```python
from build123d import *

# Parameters (mm, degrees)
SKETCH1_W           = 175
SKETCH1_H           = 150
BOSS_EXTRUDE1_DEPTH = 15
CUT_EXTRUDE1_DEPTH  = 231.976189249
SKETCH3_W           = 50
SKETCH3_H           = 30
BOSS_EXTRUDE2_DEPTH = 50
SKETCH4_W           = 40.3
SKETCH4_H           = 20.3
BOSS_EXTRUDE3_DEPTH = 25
SKETCH5_R           = 5
CUT_EXTRUDE3_DEPTH  = 206.184770127
SKETCH7_R           = 6
CUT_EXTRUDE5_DEPTH  = 248.25951426
SKETCH8_R           = 12.5
CUT_EXTRUDE6_DEPTH  = 12.5


with BuildPart() as part:
    # Sketch1 → Boss-Extrude1 (new body)
    with BuildSketch(Plane(origin=(0, 0, 0), x_dir=(1, 0, 0), z_dir=(0, 1, 0))):
        with Locations((87.5, 75)):
            Rectangle(SKETCH1_W, SKETCH1_H)
    extrude(amount=BOSS_EXTRUDE1_DEPTH)

    # Sketch2 → Cut-Extrude1 (cut, through all)
    with BuildSketch(Plane(origin=(175, 0, 0), x_dir=(0, 0, -1), z_dir=(1, 0, 0))):
        Polygon((150, 15), (0, 5), (0, 15), align=None)
    extrude(amount=-CUT_EXTRUDE1_DEPTH, mode=Mode.SUBTRACT)

    # Sketch3 → Boss-Extrude2 (add)
    with BuildSketch(Plane(origin=(0, 4.977876106, 0.331858407), x_dir=(1, 0, 0), z_dir=(0, 0.997785157856609, 0.06651901052377394))):
        with Locations((87.5, 135.665558836)):
            Rectangle(SKETCH3_W, SKETCH3_H)
    extrude(amount=BOSS_EXTRUDE2_DEPTH)

    # Sketch4 → Boss-Extrude3 (add)
    with BuildSketch(Plane(origin=(0, 54.867133999, 3.657808933), x_dir=(1, 0, 0), z_dir=(0, 0.997785157856609, 0.0665190105237739))):
        with Locations((87.5, 135.665558836)):
            Rectangle(SKETCH4_W, SKETCH4_H)
    extrude(amount=BOSS_EXTRUDE3_DEPTH)

    # Sketch5 → Cut-Extrude3 (cut, through all)
    with BuildSketch(Plane.ZY.offset(-67.35)):
        with Locations((-130.875784474, 76.363787208)):
            Circle(SKETCH5_R)
    extrude(amount=-CUT_EXTRUDE3_DEPTH, mode=Mode.SUBTRACT)

    # Sketch7 → Cut-Extrude5 (cut, through all)
    with BuildSketch(Plane.XZ):
        with Locations(Location((87.5, -131.674049474, 0), (0, 0, 270))):
            Circle(SKETCH7_R)
    extrude(amount=-CUT_EXTRUDE5_DEPTH, mode=Mode.SUBTRACT)

    # Sketch8 → Cut-Extrude6 (cut)
    with BuildSketch(Plane.XZ):
        with Locations(Location((87.5, -131.674049474, 0), (0, 0, 270))):
            Circle(SKETCH8_R)
    extrude(amount=-CUT_EXTRUDE6_DEPTH, mode=Mode.SUBTRACT)


solid = part.part
```
CAD build for the part. Positions are in the model's coordinates, mm. A direction names the side the tool comes from. Coordinates: 2 decimals unless noted, no trailing zeros. Write each loop counter-clockwise with the first axis right and the second up, starting at its lowest first coordinate (ties: lowest second). Pieces come first, ordered by that corner, then holes. Notation, with made-up numbers: (74.25, -17) -> (110.25, -17) arc R17 ccw to (110.25, 9) -> close; hole circle Ø5 at (-8, -34). An arc over 180 degrees is marked (long way). Return JSON: item names as keys, results as strings. Group by question number.
Q1. Cut at C-C, the plane z = -86. Give the cut face in (x, y), then the cut area to 3 significant figures.
Q2. Drill centre lines: line 1 (X direction, y = 41, z = -121); line 2 (X direction, y = 51, z = -127.5); line 3 (Y direction, x = 144, z = -82.5). Where is each one in solid material? Low to high.
Q3. Which spindle directions (+Z, -Z, +X, -X, +Y, -Y) get a long thin tool onto all of the face, cutting with end or side? Do faces 4 (the face through (82.1, 12.5, -128.7)), 5 (the face through (100.28, 77.87, -126.11)), 6 (the face through (87.15, 37.6, -118.427)). Say none if no direction does.
Q4. Flat gauge pins, fed straight in: pin 1 (6 mm diameter, centred on x = 21, z = -44.5, fed in from +Y); pin 2 (6.5 mm diameter, centred on y = 81.5, z = -127, fed in from -X); pin 3 (12 mm diameter, centred on x = 114.5, y = 67, fed in from +Z); pin 4 (7.5 mm diameter, centred on x = 87, z = -130, fed in from -Y). Where does each tip first touch, or does it go through?
Q5. Cut at A-A, the plane y = 28. Give the cut face in (x, z).
Q6. Pull direction X, two halves, no side cores. Call faces 1 (the face through (87.218, 76.864, -141.015)), 2 (the face through (0, 6, -91)), 3 (the face through (89.302, 50.384, -137.397)): released by +X, released by -X, zero draft, split by the parting line, or undercut.
Q7. Cut at B-B, the plane x = 13. Give the cut face in (y, z).
Returned:
{
 "1": {"outline": "(0, 0) -> (175, 0) -> (175, 10.73) -> (0, 10.73) -> close", "area": "1,880 mm2"},
 "2": {"line 1": "x = 62.5 to 112.5", "line 2": "x = 62.5 to 83.19, 91.81 to 112.5", "line 3": "y = 0 to 10.5"},
 "3": {"face 4": "-Y", "face 5": "+X, -X", "face 6": "+Z, +X, -X"},
 "4": {"pin 1": "stops at y = 8.17", "pin 2": "stops at x = 67.35", "pin 3": "stops at z = -116.74", "pin 4": "passes through"},
 "5": {"outline": "(62.5, -149.13) -> (112.5, -149.13) -> (112.5, -119.07) -> (62.5, -119.07) -> close; hole circle Ø12 at (87.5, -131.67)"},
 "6": {"face 1": "zero draft", "face 2": "released by -X", "face 3": "undercut"},
 "7": {"outline": "(0, -150) -> (15, -150) -> (5, 0) -> (0, 0) -> close"}
}
